Verification items for the finished model (mm, model axes). A direction names the side the tool comes from. Coordinates: 2 decimals unless noted, no trailing zeros. Order: outer loops, then holes, each group sorted by start corner. A loop starts at its lowest first (then second) coordinate and runs counter-clockwise, first axis right, second up. Notation, with made-up numbers: M 17.5,52.5 L 61.5,52.5 A19 cw 61.5,76.5 Z; hole C 26,77.5 d9. An arc over 180 degrees is marked long. Return JSON: item names as keys, results as strings. Group by question number.
1. Gauge pin test, flat ends, axial feed: pin 1 (1.6 mm diameter, centred on y = 2.5, z = 0, fed in from +X); pin 2 (2 mm diameter, centred on x = 13, y = -8, fed in from -Z); pin 3 (2 mm diameter, centred on x = 18.5, z = 1, fed in from -Y); pin 4 (1 mm diameter, centred on x = 9, z = -9, fed in from +Y). Record the tip position at first contact, or that the pin passes through.
2. Section check B-B, the plane y = 0. Record the cut outline in (x, z).
3. Section check C-C, the plane x = 20. Record the cut outline in (y, z).
4. Set-up check for faces 1 (the flat face through (26.5, 0, 0)), 2 (the flat face through (18, -1, 3)), 3 (the flat face through (19.5, 2, 0)): record each of +Z, -Z, +X, -X, +Y, -Y from which the full face is reachable in a straight line by a thin tool's end or side.
5. Material ranges on line 1 along X through (y, z) = (-7, -2.25); line 2 along Y through (x, z) = (9.25, 9.75); line 3 along X through (y, z) = (4.25, 4.25), recorded low to high.
6. Section check D-D, the plane y = -6. Record the cut outline in (x, z), plus the area to 3 significant figures.
7. Section check A-A, the plane z = 0. Record the cut outline in (x, y), plus the area to 3 significant figures.
```python
from build123d import *

# Parameters (mm, degrees)
CUT_EXTRUDE1_DEPTH = 7


with BuildPart() as part:
    # Sketch1 → Revolve1 (revolve)
    with BuildSketch(Plane.XY):
        Polygon((0, 0), (26.5, 0), (26.5, 3), (18, 3), (18, 4), (11.5, 4), (11.5, 7), (10.063118771, 7), (10.063118771, 12), (0, 12), align=None)
    revolve(axis=Axis((0, 0, 0), (1, 0, 0)))

    # Sketch2 → Cut-Extrude1 (cut)
    with BuildSketch(Plane(origin=(26.5, 0, 0), x_dir=(0, 0, -1), z_dir=(1, 0, 0))):
        with BuildLine():
            Line((-2.598076211, 1.5), (2.598076211, 1.5))
            ThreePointArc((2.598076211, 1.5), (0, 3), (-2.598076211, 1.5))
        make_face()
    extrude(amount=-CUT_EXTRUDE1_DEPTH, mode=Mode.SUBTRACT)


solid = part.part
```
Answers follow:
{
 "1": {"pin 1": "x = 19.5", "pin 2": "through", "pin 3": "y = -4", "pin 4": "y = 8.47"},
 "2": {"outline": "M 0,-12 L 10.06,-12 L 10.06,-7 L 11.5,-7 L 11.5,-4 L 18,-4 L 18,-3 L 26.5,-3 L 26.5,3 L 18,3 L 18,4 L 11.5,4 L 11.5,7 L 10.06,7 L 10.06,12 L 0,12 Z"},
 "3": {"outline": "M 1.5,-2.6 L 1.5,2.6 A3 ccw long Z"},
 "4": {"face 1": "+Z, -Z, +X, +Y, -Y", "face 2": "+X", "face 3": "+Z, -Z, +X, +Y"},
 "5": {"line 1": "0 to 10.06", "line 2": "-7 to 7", "line 3": "0 to 11.5"},
 "6": {"outline": "M 0,-10.39 L 10.06,-10.39 L 10.06,-3.61 L 11.5,-3.61 L 11.5,3.61 L 10.06,3.61 L 10.06,10.39 L 0,10.39 Z", "area": "220 mm^2"},
 "7": {"outline": "M 0,-12 L 10.06,-12 L 10.06,-7 L 11.5,-7 L 11.5,-4 L 18,-4 L 18,-3 L 26.5,-3 L 26.5,1.5 L 19.5,1.5 L 19.5,3 L 18,3 L 18,4 L 11.5,4 L 11.5,7 L 10.06,7 L 10.06,12 L 0,12 Z", "area": "354 mm^2"}
}
